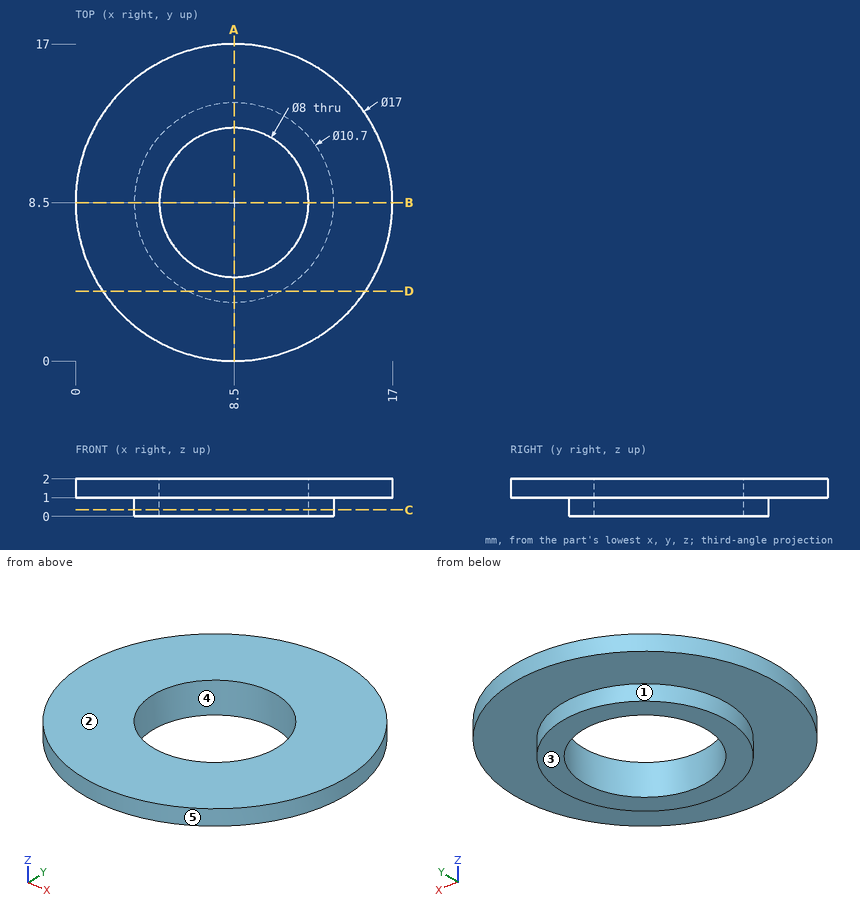
Geometry check sheet. Reference: drawing and pictorial views, mm from the part's lowest x, y, z. A direction names the side the tool comes from. Round coordinates to 2 decimals unless told otherwise and drop trailing zeros. Loops run counter-clockwise (first coordinate to the right, second up) from the corner with the lowest first, then second, coordinate; pieces in that order, holes last. Notation, with made-up numbers: (25.25, -13.5) - (81.25, -13.5) arc R11 ccw to (81.25, -1.5) - close; hole circle Ø6 at (-39.75, -31.75). An arc over 180 degrees is marked (long way). Use a Markdown table: item, result. Add a question column.
1. Access from +Z, -Z, +X, -X, +Y, -Y to the whole of each face (thin tool, end or side, straight path). Record for the marked faces 1 and 2.
2. Thickness scan on probe 1 along Y at (x, z) = (8.5, 1.25); probe 2 along Y at (x, z) = (8.5, 0.85); probe 3 along Z at (x, y) = (11, 14.75). Record the ranges inside material, lowest first. Write a range as [from, to].
3. Section check D-D, the plane y = 3.75. Record the boundary of the cut face in (x, z).
4. Release check for a two-part mould opening along Y. For the marked faces 3, 4 and 5 record: released by +Y, released by -Y, zero draft, split by the parting line, or undercut.
5. Section check A-A, the plane x = 8.5. Record the boundary of the cut face in (y, z), plus the area to 3 significant figures.
6. Section check C-C, the plane z = 0.35. Record the boundary of the cut face in (x, y), plus the area to 3 significant figures.
Checks:
| question | item | result |
|---|---|---|
| 1 | face 1 | -Z |
| 1 | face 2 | +Z, +X, -X, +Y, -Y |
| 2 | probe 1 | y = [0, 4.5], [12.5, 17] |
| 2 | probe 2 | y = [3.15, 4.5], [12.5, 13.85] |
| 2 | probe 3 | z = [1, 2] |
| 3 | outline | (1.45, 1) - (6.04, 1) - (6.04, 0) - (10.96, 0) - (10.96, 1) - (15.55, 1) - (15.55, 2) - (1.45, 2) - close |
| 4 | face 3 | zero draft |
| 4 | face 4 | undercut |
| 4 | face 5 | split by the parting line |
| 5 | outline | (0, 1) - (3.15, 1) - (3.15, 0) - (4.5, 0) - (4.5, 2) - (0, 2) - close; (12.5, 0) - (13.85, 0) - (13.85, 1) - (17, 1) - (17, 2) - (12.5, 2) - close |
| 5 | area | 11.7 mm^2 |
| 6 | outline | circle Ø10.7 at (8.5, 8.5); hole circle Ø8 at (8.5, 8.5) |
| 6 | area | 39.7 mm^2 |
